```python
from build123d import *

# Parameters (mm, degrees)
F0_R     = 2
F1_DEPTH = 4
F2_DEPTH = 7


# Not quite as in the source:
# - a feature names something its author has since deleted; it is built from what else it names


with BuildPart() as f1:
    # F0 (on Top) → F1 (new body)
    with BuildSketch(Plane.XY):
        with BuildLine():
            ThreePointArc((8.8045736775, 5.9720319696), (4.7714301194, 13.5077650507), (-3.2184339135, 10.47204557))
            ThreePointArc((-3.2184339135, 10.47204557), (-7.0349525259, 0.086158841), (-4.7456540833, -10.739346695))
            ThreePointArc((-4.7456540833, -10.739346695), (-0.5751322141, -13.8008387314), (4.5426217839, -13.0428280681))
            ThreePointArc((4.5426217839, -13.0428280681), (5.4021565515, -3.2504198201), (8.8045736775, 5.9720319696))
        make_face()
        with Locations((1.0620787063, -7.3684426025)):
            Circle(F0_R, mode=Mode.SUBTRACT)
        with Locations((2.5027735673, 7.4464333818)):
            Circle(F0_R, mode=Mode.SUBTRACT)
    extrude(amount=-F1_DEPTH)

    # F0 (on Top) → F2 (join)
    with BuildSketch(Plane.XY):
        with Locations((2.5027735673, 7.4464333818)):
            Circle(F0_R)
        with Locations((1.0620787063, -7.3684426025)):
            Circle(F0_R)
    extrude(amount=-F2_DEPTH)


solid = f1.part
```
Check sheet for the modelled part. Datum: model origin and axes. Units: mm. A direction names the side the tool comes from. Round coordinates to 2 decimals unless told otherwise and drop trailing zeros. Loops run counter-clockwise (first coordinate to the right, second up) from the corner with the lowest first, then second, coordinate; pieces in that order, holes last. Notation, with made-up numbers: (-17, -16.5) - (10, -16.5) arc R28 ccw to (10, 3.5) - close; hole circle Ø4 at (18, 53). An arc over 180 degrees is marked (long way). Answer as a JSON object with one key per item and string values. Group by question number.
Q1. Sectioned sample at D-D, the plane z = -3. Enter the section's corners in (x, y), plus the area to 3 significant figures.
Q2. Gauge pin test, flat ends, axial feed: P1, Ø1, axis at x = 5.5, y = 2, coming from the -Z side; P2, Ø3, axis at x = -4.5, z = -1, coming from the -Y side. Record the tip position at first contact, or that the pin passes through.
Q3. Set-up check for faces 5 (the face through (1, 0, -4)), 6 (the face through (1, 0, 0)), 7 (the face through (5.37, -3.39, -1.97)): record each of +Z, -Z, +X, -X, +Y, -Y from which the full face is reachable in a straight line by a thin tool's end or side.
Q4. Sectioned sample at C-C, the plane z = -4.75. Enter the section's corners in (x, y).
Q5. Sectioned sample at B-B, the plane y = -6.25. Enter the section's corners in (x, z), plus the area to 3 significant figures.
Q6. Mould release check, pull along Y, two halves, no side actions. Record for faces 1 (the face through (2, 7, -7)), 2 (the face through (-7.023, 0.243, -1.972)), 3 (the face through (2.24, 9.43, -5.48)), 4 (the face through (-0.65, -13.78, -1.97)): released by +Y, released by -Y, zero draft, split by the parting line, or undercut.
Q7. Scan lines: line 1 along Z through (x, y) = (-3, -10.5); line 2 along Y through (x, z) = (1.75, -4.25); line 3 along Y through (x, z) = (1, -6.25). Record each from-to range of solid material in increasing order. Write a range as [from, to].
Q8. Sectioned sample at A-A, the plane x = 1.5. Enter the section's corners in (y, z), plus the area to 3 significant figures.
Solution:
{
 "1": {"outline": "(-4.75, -10.74) arc R6.8 ccw to (4.54, -13.04) arc R37.08 cw to (8.8, 5.97) arc R6.47 ccw to (-3.22, 10.47) arc R20 ccw to start", "area": "319 mm²"},
 "2": {"P1": "stops at z = -4", "P2": "stops at y = -12.65"},
 "3": {"face 5": "-Z", "face 6": "+Z, +X, -X, +Y, -Y", "face 7": "+Z, -Z, +X"},
 "4": {"outline": "circle Ø4 at (1.06, -7.37); circle Ø4 at (2.5, 7.45)"},
 "5": {"outline": "(-6.48, -4) - (-0.6, -4) - (-0.6, -7) - (2.72, -7) - (2.72, -4) - (4.86, -4) - (4.86, 0) - (-6.48, 0) - close", "area": "55.3 mm²"},
 "6": {"face 1": "zero draft", "face 2": "split by the parting line", "face 3": "undercut", "face 4": "released by -Y"},
 "7": {"line 1": "z = [-4, 0]", "line 2": "y = [-9.25, -5.49], [5.59, 9.3]", "line 3": "y = [-9.37, -5.37], [6.13, 8.77]"},
 "8": {"outline": "(-13.99, -4) - (-9.32, -4) - (-9.32, -7) - (-5.42, -7) - (-5.42, -4) - (5.72, -4) - (5.72, -7) - (9.18, -7) - (9.18, -4) - (13.84, -4) - (13.84, 0) - (-13.99, 0) - close", "area": "133 mm²"}
}
